Source: CAD feature listing. Evaluate the final solid. Frame: model axes, mm. Coordinates: 2 decimals unless noted, no trailing zeros. Write each loop counter-clockwise with the first axis right and the second up, starting at its lowest first coordinate (ties: lowest second). Pieces come first, ordered by that corner, then holes. Notation, with made-up numbers: (-10, 2) - (45, 2) arc R23 cw to (45, 13) - close; hole circle Ø4 at (42, 74.25). An arc over 180 degrees is marked (long way). One line per question, with ' | ' between items.
from build123d import *

# Parameters (mm, degrees)
MODEL_R             = 1.500000002
MODEL_R_2           = 1.35
MODEL_R_3           = 1.500000003
MODEL_W             = 3
MODEL_H             = 10
BOSS_EXTRUDE1_DEPTH = 3


with BuildPart() as part:
    # Model → Boss-Extrude1 (new body)
    with BuildSketch(Plane.XY):
        with BuildLine():
            Line((77.350374728, 38.932799758), (77.3504385, 61.847914879))
            ThreePointArc((77.3504385, 61.847914879), (76.471798677, 63.969197152), (74.350545547, 64.84790733))
            Line((74.350545547, 64.84790733), (73.850545547, 64.84790733))
            Line((73.850545547, 64.84790733), (20.350545547, 64.848184253))
            ThreePointArc((20.350545547, 64.848184253), (18.229231749, 63.96968584), (17.350530152, 61.848456197))
            Line((17.350530152, 61.848456197), (17.350325984, 19.035510771))
            Line((17.350325984, 19.035510771), (17.350321434, 18.148199638))
            ThreePointArc((17.350321434, 18.148199638), (18.228860554, 16.026745133), (20.350306049, 15.148184254))
            Line((20.350306049, 15.148184254), (32.850606049, 15.14812015))
            Line((32.850606049, 15.14812015), (74.350306048, 15.147907331))
            ThreePointArc((74.350306048, 15.147907331), (76.471660555, 16.026546451), (77.350321433, 18.147891946))
            Line((77.350321433, 18.147891946), (77.350374728, 38.932799758))
        make_face()
        with Locations((47.350513739, 55.648045793)):
            Circle(MODEL_R, mode=Mode.SUBTRACT)
        with Locations((37.850318867, 18.148094512)):
            Circle(MODEL_R_2, mode=Mode.SUBTRACT)
        with Locations((37.850416303, 36.148094512)):
            Circle(MODEL_R_2, mode=Mode.SUBTRACT)
        with Locations((21.850472716, 47.648176561)):
            Circle(MODEL_R_3, mode=Mode.SUBTRACT)
        Polygon((23.350454767, 44.148168869), (23.350423998, 38.148168869), (20.350423998, 38.148184254), (20.350454767, 44.148184254), align=None, mode=Mode.SUBTRACT)
        Polygon((23.350521434, 57.148168869), (23.350490665, 51.148168869), (20.350490665, 51.148184253), (20.350521434, 57.148184253), align=None, mode=Mode.SUBTRACT)
        Polygon((49.350336818, 21.148035536), (49.350398356, 33.148035536), (26.350398357, 33.148153484), (26.350336818, 21.148153485), align=None, mode=Mode.SUBTRACT)
        Polygon((34.850506049, 54.148109894), (34.850521434, 57.148109894), (24.850521434, 57.148161176), (24.850506049, 54.148161176), align=None, mode=Mode.SUBTRACT)
        Polygon((69.850505905, 54.147930167), (69.850521433, 57.147930167), (59.850505905, 57.147981929), (59.850505905, 54.147930167), align=None, mode=Mode.SUBTRACT)
        with Locations((68.28527947, 30.147930167)):
            Rectangle(MODEL_W, MODEL_H, mode=Mode.SUBTRACT)
    extrude(amount=BOSS_EXTRUDE1_DEPTH)


solid = part.part
Item 1: Cut plane A-A on x = 40.5. Return loops of the section in (y, z), and give its area (3 significant figures).
Check sheet entries:
outline: (15.15, 0) - (21.15, 0) - (21.15, 3) - (15.15, 3) - close; (33.15, 0) - (64.85, 0) - (64.85, 3) - (33.15, 3) - close | area: 113 mm²
Item 2: Cut plane D-D on z = 2.4. State how many separate pieces and enclosed holes the cut face has, and give its area (3 significant figures).
Check sheet entries:
separate pieces: 1 | enclosed holes: 10 | area: 2,550 mm²
Item 3: Cut plane C-C on x = 22.5. Return loops of the section in (y, z).
Check sheet entries:
outline: (15.15, 0) - (38.15, 0) - (38.15, 3) - (15.15, 3) - close; (44.15, 0) - (46.3, 0) - (46.3, 3) - (44.15, 3) - close; (49, 0) - (51.15, 0) - (51.15, 3) - (49, 3) - close; (57.15, 0) - (64.85, 0) - (64.85, 3) - (57.15, 3) - close
Item 4: Cut plane B-B on y = 40.5. Return loops of the section in (x, z).
Check sheet entries:
outline: (17.35, 0) - (20.35, 0) - (20.35, 3) - (17.35, 3) - close; (23.35, 0) - (77.35, 0) - (77.35, 3) - (23.35, 3) - close
Item 5: Pin query (flat end, axial travel): pin 1 Ø4 at (x, y) = (21.85, 47.65) entering from -Z. Return the tip coordinate at first contact, or that it passes through.
Check sheet entries:
pin 1: z = 0
Item 6: Mould query, pull axis X, two halves, no side actions, for faces 1 (the face through (68, 25.148, 1)), 2 (the face through (18.25, 63.99, 1.48)), 3 (the face through (76.49, 63.95, 1.48)). Classes: pulls with the +X half, pulls with the -X half, needs draft (parallel to the pull), parting line crosses it, or undercut.
Check sheet entries:
face 1: undercut | face 2: pulls with the -X half | face 3: pulls with the +X half
Item 7: Ray query, line 1 along Y through (x, z) = (33.5, 2.25); line 2 along X through (y, z) = (30, 2.8); line 3 along X through (y, z) = (40.5, 0.9). Return the intervals inside material, ascending. Write a range as [from, to].
Check sheet entries:
line 1: [15.15, 21.15], [33.15, 54.15], [57.15, 64.85] | line 2: [17.35, 26.35], [49.35, 66.79], [69.79, 77.35] | line 3: [17.35, 20.35], [23.35, 77.35]
